Verification items for the finished model (mm, model axes). Face numbers are marked on the shaded views. A direction names the side the tool comes from. Give positions to 0.01 mm unless a question says otherwise; leave off trailing zeros. Order: outer loops, then holes, each group sorted by start corner. A loop starts at its lowest first (then second) coordinate and runs counter-clockwise, first axis right, second up. Notation, with made-up numbers: (16.5, 45) -> (25.5, 45) arc R23 cw to (25.5, 60) -> close; hole circle Ø2 at (5.5, 70.25). An arc over 180 degrees is marked (long way). One line per question, with ' | ' between items. Start each with the question number.
Q1. Section check C-C on y = 41. Record the cut outline in (x, z), plus the area to 3 significant figures.
Q2. Section check B-B on x = 16. Record the cut outline in (y, z).
Q3. Mould release check, pull along Y, two halves, no side actions. Record for the marked faces 5, 6 and 7: released by +Y, released by -Y, zero draft, split by the parting line, or undercut.
Q4. Material ranges on probe 1 along Z at (x, y) = (10.5, 25.5); probe 2 along Y at (x, z) = (15, 7), recorded low to high. Write a range as [from, to].
Q5. Section check A-A on z = -0.5. Record the cut outline in (x, y).
Q6. Section check D-D on y = 27.5. Record the cut outline in (x, z), plus the area to 3 significant figures.
Q7. Go/stop test with flat-tipped pins: pin 1 (2 mm diameter, centred on y = 38.5, z = 15.5, fed in from -X); pin 2 (10 mm diameter, centred on y = 39, z = -0.5, fed in from +X) (3 decimals); pin 3 (8 mm diameter, centred on x = -13, y = 10.5, fed in from +Z). Record where each tip stops, or that it passes through.
Q8. Access from +Z, -Z, +X, -X, +Y, -Y to the whole of each face (thin tool, end or side, straight path). Record for the marked faces 1, 2, 3 and 4.
from build123d import *

# Parameters (mm, degrees)
BOSS_EXTRUDE1_DEPTH = 26
BOSS_EXTRUDE2_DEPTH = 20
RIB1_REACH          = 65.39
SKETCH6_WALL_W      = 172.439958848
SKETCH6_WALL_H      = 8
RIB2_REACH          = 65.39
SKETCH7_WALL_W      = 172.439958848
SKETCH7_WALL_H      = 8


with BuildPart() as part:
    # Sketch2 → Boss-Extrude1 (new, symmetric)
    with BuildSketch(Plane.XY):
        Polygon((-5, 4), (37.5, 4), (37.5, -4), (-37.5, -4), (-37.5, 4), align=None)
    extrude(amount=BOSS_EXTRUDE1_DEPTH, both=True)

    # Sketch2<3> → Boss-Extrude2 (add, symmetric)
    with BuildSketch(Plane.XY):
        with BuildLine():
            Line((-5, 24.635083269), (-5, 4))
            Line((-5, 4), (5, 4))
            Line((5, 4), (5, 24.635083269))
            ThreePointArc((5, 24.635083269), (15.811388301, 31.752551286), (20, 44))
            Line((20, 44), (12, 44))
            ThreePointArc((12, 44), (0, 32), (-12, 44))
            Line((-12, 44), (-20, 44))
            ThreePointArc((-20, 44), (-15.811388301, 31.752551286), (-5, 24.635083269))
        make_face()
    extrude(amount=BOSS_EXTRUDE2_DEPTH, both=True)

    # Sketch6 wall → Rib1 (add, up to next)
    with BuildSketch(Plane(origin=(28.75, 24, 0), x_dir=(0.40081883402, -0.916157334902, 0), z_dir=(0.916157334902, 0.40081883402, 0)), mode=Mode.PRIVATE) as rib1_sk1:
        Rectangle(SKETCH6_WALL_W, SKETCH6_WALL_H)
    rib1_tool1 = extrude(rib1_sk1.sketch, amount=-RIB1_REACH, mode=Mode.PRIVATE) - part.part
    add(rib1_tool1.solids().sort_by_distance((28.75, 24, 0))[0])

    # Sketch7 wall → Rib2 (add, up to next)
    with BuildSketch(Plane(origin=(-28.75, 24, 0), x_dir=(-0.40081883402, -0.916157334902, 0), z_dir=(0.916157334902, -0.40081883402, 0)), mode=Mode.PRIVATE) as rib2_sk1:
        Rectangle(SKETCH7_WALL_W, SKETCH7_WALL_H)
    rib2_tool1 = extrude(rib2_sk1.sketch, amount=RIB2_REACH, mode=Mode.PRIVATE) - part.part
    add(rib2_tool1.solids().sort_by_distance((-28.75, 24, 0))[0])


solid = part.part
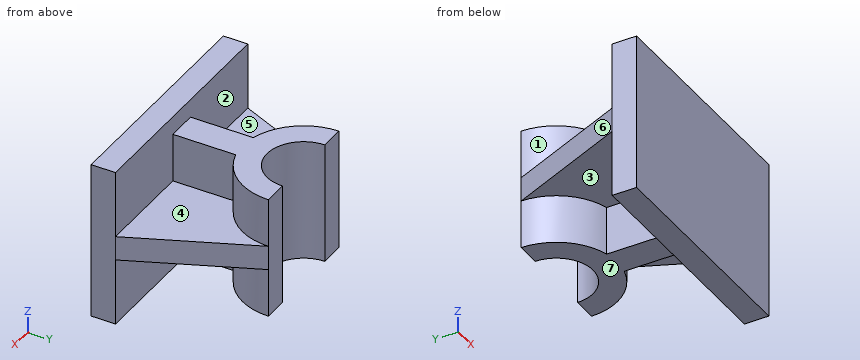
Filled in:
1) outline: (-21.31, -4) -> (-19.77, -4) -> (-19.77, -20) -> (-11.62, -20) -> (-11.62, 20) -> (-19.77, 20) -> (-19.77, 4) -> (-21.31, 4) -> close; (11.62, -20) -> (19.77, -20) -> (19.77, -4) -> (21.31, -4) -> (21.31, 4) -> (19.77, 4) -> (19.77, 20) -> (11.62, 20) -> close | area: 677 mm²
2) outline: (-4, -26) -> (4, -26) -> (4, -4) -> (32, -4) -> (32, -20) -> (44, -20) -> (44, 20) -> (32, 20) -> (32, 4) -> (4, 4) -> (4, 26) -> (-4, 26) -> close
3) face 5: undercut | face 6: released by +Y | face 7: zero draft
4) probe 1: [-4, 4] | probe 2: [-4, 4], [30.77, 44]
5) outline: (-37.5, -4) -> (37.5, -4) -> (37.5, 4) -> (20, 44) -> (12, 44) arc R12 cw to (-12, 44) -> (-20, 44) -> (-37.5, 4) -> close
6) outline: (-27.22, -4) -> (-11.3, -4) -> (-11.3, -20) -> (11.3, -20) -> (11.3, -4) -> (27.22, -4) -> (27.22, 4) -> (11.3, 4) -> (11.3, 20) -> (-11.3, 20) -> (-11.3, 4) -> (-27.22, 4) -> close | area: 1,160 mm²
7) pin 1: x = -19.49 | pin 2: x = 24.375 | pin 3: z = 4
8) face 1: +Z, -X | face 2: +Z | face 3: -Z, -X | face 4: +Z, +X
